from build123d import *
from build123d.topology import SkipClean

# Parameters (mm, degrees)
BOSS_EXTRUDE1_DEPTH = 11.176
CUT_EXTRUDE3_DEPTH  = 145.042188445
SKETCH2_4_R         = 16.51
SKETCH2_4_R_2       = 6.35
BOSS_EXTRUDE2_DEPTH = 25.4
SKETCH3_R           = 0.635
CUT_EXTRUDE4_DEPTH  = 119.599506053
CUT_EXTRUDE5_DEPTH  = 146.259799711
BOSS_EXTRUDE3_DEPTH = 25.4
FILLET5_R           = 2.54
FILLET6_R           = 19.05
FILLET9_R           = 12.7


with BuildPart() as part:
    # Sketch1 → Boss-Extrude1 (new, symmetric)
    with BuildSketch(Plane.XY):
        with BuildLine():
            Line((-23.876, -12.7), (-23.876, 57.15))
            Line((-23.876, 57.15), (-17.526, 57.15))
            ThreePointArc((-17.526, 57.15), (-13.035871939, 55.290128061), (-11.176, 50.8))
            Line((-11.176, 50.8), (-11.176, 36.576))
            ThreePointArc((-11.176, 36.576), (0, 25.4), (11.176, 36.576))
            Line((11.176, 36.576), (11.176, 50.8))
            ThreePointArc((11.176, 50.8), (13.035871939, 55.290128061), (17.526, 57.15))
            Line((17.526, 57.15), (23.876, 57.15))
            Line((23.876, 57.15), (23.876, 12.7))
            Line((23.876, 12.7), (125.476, 12.7))
            Line((125.476, 12.7), (125.476, -12.7))
            Line((125.476, -12.7), (-23.876, -12.7))
        make_face()
    extrude(amount=BOSS_EXTRUDE1_DEPTH, both=True)

    # Sketch2 → Cut-Extrude3 (cut, through all)
    with BuildSketch(Plane(origin=(0, -12.7, 0), x_dir=(-1, 0, 0), z_dir=(0, -1, 0))):
        with BuildLine():
            ThreePointArc((-124.4078631, -11.176), (-125.206770606, -8.303422521), (-125.476, -5.334))
            Line((-125.476, -5.334), (-125.476, -11.176))
            Line((-125.476, -11.176), (-124.4078631, -11.176))
        make_face()
        with BuildLine():
            ThreePointArc((-106.477318421, -11.176), (-108.966, 1.016), (-111.454681579, -11.176))
            Line((-111.454681579, -11.176), (-106.477318421, -11.176))
        make_face()
    extrude(amount=-CUT_EXTRUDE3_DEPTH, mode=Mode.SUBTRACT)

    # Sketch2<4> → Boss-Extrude2 (add)
    with SkipClean():  # the faces are left unmerged after this step: merging them gives an invalid solid
        with BuildSketch(Plane(origin=(0, -12.7, 0), x_dir=(-1, 0, 0), z_dir=(0, -1, 0))):
            with Locations((-108.966, -5.334)):
                Circle(SKETCH2_4_R)
            with Locations(Location((-108.966, -5.334, 0), (0, 0, 180))):
                Circle(SKETCH2_4_R_2, mode=Mode.SUBTRACT)
        extrude(amount=-BOSS_EXTRUDE2_DEPTH)

    # Sketch3 → Cut-Extrude4 (cut, through all)
    with SkipClean():  # the faces are left unmerged after this step: merging them gives an invalid solid
        with BuildSketch(Plane(origin=(23.876, 0, 0), x_dir=(0, 0, -1), z_dir=(1, 0, 0))):
            with Locations((6.35, 22.225)):
                Circle(SKETCH3_R)
            with Locations(Location((-6.35, 22.225, 0), (0, 0, 180))):
                Circle(SKETCH3_R)
            with Locations(Location((6.35, 47.625, 0), (0, 0, 270))):
                Circle(SKETCH3_R)
            with Locations((-6.35, 47.625)):
                Circle(SKETCH3_R)
        extrude(amount=-CUT_EXTRUDE4_DEPTH, mode=Mode.SUBTRACT)

    # Sketch4 → Cut-Extrude5 (cut, through all)
    with SkipClean():  # the faces are left unmerged after this step: merging them gives an invalid solid
        with BuildSketch(Plane(origin=(0, -12.7, 0), x_dir=(-1, 0, 0), z_dir=(0, -1, 0))):
            with BuildLine():
                Line((-59.436, -7.366), (-59.436, -11.176))
                Line((-59.436, -11.176), (-53.086, -11.176))
                ThreePointArc((-53.086, -11.176), (-54.201923164, -8.481923164), (-56.896, -7.366))
                Line((-56.896, -7.366), (-59.436, -7.366))
            make_face()
            with BuildLine():
                Line((-70.866, -11.176), (-64.516, -11.176))
                Line((-64.516, -11.176), (-64.516, -7.366))
                Line((-64.516, -7.366), (-67.056, -7.366))
                ThreePointArc((-67.056, -7.366), (-69.750076836, -8.481923164), (-70.866, -11.176))
            make_face()
            with BuildLine():
                Line((-59.436, -11.176), (-59.436, -14.986))
                Line((-59.436, -14.986), (-56.896, -14.986))
                ThreePointArc((-56.896, -14.986), (-54.201923164, -13.870076836), (-53.086, -11.176))
                Line((-53.086, -11.176), (-59.436, -11.176))
            make_face()
            with BuildLine():
                Line((-64.516, -14.986), (-64.516, -11.176))
                Line((-64.516, -11.176), (-70.866, -11.176))
                ThreePointArc((-70.866, -11.176), (-69.750076836, -13.870076836), (-67.056, -14.986))
                Line((-67.056, -14.986), (-64.516, -14.986))
            make_face()
        extrude(amount=-CUT_EXTRUDE5_DEPTH, mode=Mode.SUBTRACT)

    # Sketch4<3> → Boss-Extrude3 (add)
    with SkipClean():  # the faces are left unmerged after this step: merging them gives an invalid solid
        with BuildSketch(Plane(origin=(0, -12.7, 0), x_dir=(-1, 0, 0), z_dir=(0, -1, 0))):
            with BuildLine():
                Line((-56.896, -14.986), (-59.436, -14.986))
                Line((-59.436, -14.986), (-59.436, -11.176))
                Line((-59.436, -11.176), (-64.516, -11.176))
                Line((-64.516, -11.176), (-64.516, -14.986))
                Line((-64.516, -14.986), (-67.056, -14.986))
                ThreePointArc((-67.056, -14.986), (-69.750076836, -13.870076836), (-70.866, -11.176))
                Line((-70.866, -11.176), (-84.515613398, -11.176))
                ThreePointArc((-84.515613398, -11.176), (-78.753082295, -12.558613584), (-74.245252576, -16.405411765))
                ThreePointArc((-74.245252576, -16.405411765), (-71.089771772, -19.098170491), (-67.056, -20.066))
                Line((-67.056, -20.066), (-56.896, -20.066))
                ThreePointArc((-56.896, -20.066), (-52.862228228, -19.098170491), (-49.706747424, -16.405411765))
                ThreePointArc((-49.706747424, -16.405411765), (-45.198917705, -12.558613584), (-39.436386602, -11.176))
                Line((-39.436386602, -11.176), (-53.086, -11.176))
                ThreePointArc((-53.086, -11.176), (-54.201923164, -13.870076836), (-56.896, -14.986))
            make_face()
        extrude(amount=-BOSS_EXTRUDE3_DEPTH)

    # Fillet5
    fillet5_edges = [part.edges().sort_by_distance(p)[0] for p in [
        (54.201923164, -12.7, 13.870076836),
        (54.201923164, 12.7, 8.481923164),
        (69.750076836, -12.7, 8.481923164),
        (69.750076836, 12.7, 8.481923164),
        (59.436, 0, 14.986),
        (59.436, -12.7, 13.081),
        (59.436, 12.7, 9.271),
        (64.516, 0, 14.986),
        (64.516, 12.7, 13.081),
        (64.516, -12.7, 13.081),
        (59.436, 0, 7.366),
        (64.516, 0, 7.366),
    ]]
    fillet(fillet5_edges, radius=FILLET5_R - 0.0001)  # a hair under: the kernel refuses the full size


with BuildPart() as body_2:
    # Mirror1: mirrored copy
    add(part.part.mirror(Plane(origin=(0, 0, 0), x_dir=(0, 0, 1), z_dir=(1, 0, 0))))

    # Fillet6
    fillet6_edges = [body_2.edges().sort_by_distance(p)[0] for p in [
        (23.876, -12.7, 0),
    ]]
    fillet(fillet6_edges, radius=FILLET6_R)

    # Fillet9
    fillet9_edges = [body_2.edges().sort_by_distance(p)[0] for p in [
        (-93.5241369, 0, 11.176),
    ]]
    fillet(fillet9_edges, radius=FILLET9_R)


solid = body_2.part
Geometry: final body of the model. Coordinates: model frame, mm. A direction names the side the tool comes from. Give positions to 0.01 mm unless a question says otherwise; leave off trailing zeros. Order: outer loops, then holes, each group sorted by start corner. A loop starts at its lowest first (then second) coordinate and runs counter-clockwise, first axis right, second up. Notation, with made-up numbers: (3.5, 51) -> (42.5, 51) arc R14 cw to (42.5, 63) -> close; hole circle Ø3 at (46, 59). An arc over 180 degrees is marked (long way). Answer as a JSON object with one key per item and string values.
Q1. Access query for faces 1 (the cylindrical face through (-63.75, -11.98, 11.19)), 2 (the flat face through (-75, 12.7, 1)), 3 (the cylindrical face through (-60.16, 11.936, 11.194)), 4 (the flat face through (-64.516, 0, 11)), 5 (the cylindrical face through (13.086, 55.339, 0.156)). Directions: +Z, -Z, +X, -X, +Y, -Y. A direction counts if a zero-diameter tool reaches every point of the face in a straight line with its end or side. Return the directions, or none.
Entries:
{"face 1": "-Y", "face 2": "+Z, -Z, -X, +Y", "face 3": "+Y", "face 4": "+Y, -Y", "face 5": "+Z, -Z, +Y"}
Q2. Draft query along Z for faces 6 (the cylindrical face through (-71.142, -0.178, 19.071)), 7 (the cylindrical face through (-60.16, -11.936, 11.158)), 8 (the flat face through (-35, 7, -11.176)), 9 (the cylindrical face through (18.444, -6.971, 0.156)). Return one class per face: released by +Z, released by -Z, zero draft, split by the parting line, or undercut.
Entries:
{"face 6": "released by +Z", "face 7": "undercut", "face 8": "released by -Z", "face 9": "zero draft"}
Q3. Section B-B (z = 0.5). Output: boundary loops of the cut face in (x, y), plus the area to 3 significant figures.
Entries:
{"outline": "(-125.48, -12.7) -> (-113.08, -12.7) -> (-113.08, 12.7) -> (-125.48, 12.7) -> close; (-104.85, -12.7) -> (4.83, -12.7) arc R19.05 ccw to (23.88, 6.35) -> (23.88, 57.15) -> (17.53, 57.15) arc R6.35 ccw to (11.18, 50.8) -> (11.18, 36.58) arc R11.18 cw to (-11.18, 36.58) -> (-11.18, 50.8) arc R6.35 ccw to (-17.53, 57.15) -> (-23.88, 57.15) -> (-23.88, 12.7) -> (-104.85, 12.7) -> close", "area": "4,960 mm^2"}
Q4. Section A-A (y = 42). Output: boundary loops of the cut face in (x, z), plus the area to 3 significant figures.
Entries:
{"outline": "(-23.88, -11.18) -> (-11.18, -11.18) -> (-11.18, 11.18) -> (-23.88, 11.18) -> close; (11.18, -11.18) -> (23.88, -11.18) -> (23.88, 11.18) -> (11.18, 11.18) -> close", "area": "568 mm^2"}
Q5. Section C-C (y = 8). State how many separate pieces and enclosed holes the cut face has, plus the area to 3 significant figures.
Entries:
{"separate pieces": "1", "enclosed holes": "3", "area": "3,610 mm^2"}
Q6. First-contact query: pin 1 (1.3 mm diameter, centred on y = -2, z = 10.5, fed in from +X); pin 2 (1.1 mm diameter, centred on y = 47.625, z = 6.35, fed in from -X); pin 3 (1 mm diameter, centred on y = 36, z = -7, fed in from -X); pin 4 (2 mm diameter, centred on x = -103, z = 6.5, fed in from +Y). Flat tips, straight axial feed; report the tip coordinate or a pass-through.
Entries:
{"pin 1": "stops at x = 22.25", "pin 2": "passes through", "pin 3": "stops at x = -23.88", "pin 4": "stops at y = 12.7"}
Q7. Section D-D (x = 0). Output: boundary loops of the cut face in (y, z) (3 decimals).
Entries:
{"outline": "(-12.7, -11.176) -> (25.4, -11.176) -> (25.4, 11.176) -> (-12.7, 11.176) -> close; hole circle Ø1.27 at (22.225, -6.35); hole circle Ø1.27 at (22.225, 6.35)"}
Q8. Material intervals for probe 1 along Y at (x, z) = (-18.75, -6.35); probe 2 along X at (y, z) = (50, -6.5); probe 3 along Y at (x, z) = (18, 6.35), sorted ascending.
Entries:
{"probe 1": "y = -12.7 to 21.59, 22.86 to 46.99, 48.26 to 57.15", "probe 2": "x = -23.88 to -11.18, 11.18 to 23.88", "probe 3": "y = -7.41 to 21.59, 22.86 to 46.99, 48.26 to 57.15"}
